Autodesk Fusion 360 part; units mm, degrees
sketch "Skizze2" plane through (0, 0, 0) normal (0, 0, 1) x (1, 0, 0)
  line L0 (15, 50) -> (-15, 50)
  line L1 (-15, 50) -> (-15, -50)
  line L2 (-15, -50) -> (15, -50)
  line L3 (15, -50) -> (15, 50)
  line L4 (15, 50) -> (-15, -50) construction
  line L5 (-15, 50) -> (15, -50) construction
  circle A0 centre (15, 50) radius 2.3
  circle A1 centre (-15, 50) radius 2.3
  circle A2 centre (-15, -50) radius 2.3
  circle A3 centre (15, -50) radius 2.3
  line L6 (40, 86) -> (-40, 86)
  line L7 (-40, 86) -> (-40, -86)
  line L8 (-40, -86) -> (40, -86)
  line L9 (40, -86) -> (40, 86)
  line L10 (40, 86) -> (-40, -86) construction
  line L11 (-40, 86) -> (40, -86) construction
  line L12 (-30, -86) -> (-30, 86)
  line L13 (30, 86) -> (30, -86)
  line L14 (0, 0) -> (0, -50)
  circle A4 centre (-30, -76) radius 2.75
  circle A5 centre (-30, 0) radius 2.75
  circle A6 centre (-30, 76) radius 2.75
  line L15 (-30, 76) -> (30, 76)
  line L16 (-30, 0) -> (30, 0)
  line L17 (-30, -76) -> (30, -76)
  circle A7 centre (30, -76) radius 2.75
  circle A8 centre (30, 0) radius 2.75
  circle A9 centre (30, 76) radius 2.75
  dimension "d1" = 4.6
  dimension "d2" = 30
  dimension "d3" = 100
  dimension "d4" = 36
  dimension "d5" = 80
  dimension "d6" = 60
  dimension "d7" = 10
  dimension "d8" = 10
  dimension "d9" = 5.5
extrude "Extrusion1" add sketch "Skizze2" against normal blind 6 contours L0 L1 L3 A0 A1 L12 L13 A5 A6 L15 L16 A8 A9 | L0 L1 L3 A0 A1 L16 | L1 L2 A2 L14 L16 | L1 L2 L3 A2 A3 L12 L13 A4 A5 L16 L17 A7 A8 | L2 L3 A3 L14 L16 | L6 L7 L8 L12 A4 A5 A6 | L6 L8 L9 L13 A7 A8 A9 | L6 L12 L13 A6 L15 A9 | L8 L12 L13 A4 L17 A7
fillet "Abrundung1" radius 5 4 edges at (40, -86, -3) (-40, -86, -3) (40, 86, -3) (-40, 86, -3)
hole "Bohrung1" at (30, 0, 0) at (30, 76, 0) at (30, -76, 0) at (-30, -76, 0) at (-30, 0, 0) at (-30, 76, 0) direction (0, 0, -1) diameter 5 depth 30 tip angle 118 countersink diameter 10.5 countersink angle 90
equation "d8 = d7"
Could you check a few things on this model? Use its own coordinates, in mm. Coordinates: 2 decimals unless noted, no trailing zeros. Loops run counter-clockwise (first coordinate to the right, second up) from the corner with the lowest first, then second, coordinate; pieces in that order, holes last. Notation, with made-up numbers: M 72.5,50 L 76.5,50 A16 cw 76.5,68 Z; hole C 89.25,88.5 d5. An arc over 180 degrees is marked long. Put each result on its own line as item: value. Start each with the question number.
(1) Suppose I cut it at C-C on x = 15. Please give me the cut outline in (y, z), then the cut area to 3 significant figures.
(2) I need wall thicknesses on line 1 (Y direction, x = 15, z = -1.5); line 2 (Y direction, x = 30, z = -5.2); line 3 (X direction, y = 76, z = -4.55). Which ranges of each line are inside material? Lowest first, please. Write a range as from..to.
(3) Will these pins go through, and if not, where does the flat tip stop? P1, Ø9, axis at x = 30, y = 76, coming from the +Z side; P2, Ø3, axis at x = -15, y = 50, coming from the +Z side; P3, Ø6.5, axis at x = 30, y = 0, coming from the +Z side.
(4) Suppose I cut it at A-A on y = 0. Please give me the cut outline in (x, z), then the cut area to 4 significant figures.
(5) Suppose I cut it at D-D on y = -50. Please give me the cut outline in (x, z).
(6) Suppose I cut it at B-B on z = -1.3. Count the separate pieces of the cut face and the enclosed holes in it, then the cut area to 3 significant figures.
(7) Thinking about a two-plate mould opening in X: for faces 1 (the face through (30.128, -73.096, -2.344)), 2 (the face through (-39, 84, -3)), 3 (the face through (-13.94, -52.04, -2.96)), 4 (the face through (-1, 1, 0)), which applies, pulls with the +X half, pulls with the -X half, needs draft (parallel to the pull), parting line crosses it, or undercut?
Solutions:
1. outline: M -86,-6 L -52.3,-6 L -52.3,0 L -86,0 Z; M -47.7,-6 L 47.7,-6 L 47.7,0 L -47.7,0 Z; M 52.3,-6 L 86,-6 L 86,0 L 52.3,0 Z
1. area: 977 mm2
2. line 1: y = -86..-52.3, -47.7..47.7, 52.3..86
2. line 2: y = -86..-78.75, -73.25..-2.75, 2.75..73.25, 78.75..86
2. line 3: x = -40..-32.75, -27.25..27.25, 32.75..40
3. P1: stops at z = -0.75
3. P2: passes through
3. P3: stops at z = -2
4. outline: M -40,-6 L -32.75,-6 L -32.75,-2.5 L -35.25,0 L -40,0 Z; M -27.25,-6 L 27.25,-6 L 27.25,-2.5 L 24.75,0 L -24.75,0 L -27.25,-2.5 Z; M 32.75,-6 L 40,-6 L 40,0 L 35.25,0 L 32.75,-2.5 Z
4. area: 401.5 mm2
5. outline: M -40,-6 L -17.3,-6 L -17.3,0 L -40,0 Z; M -12.7,-6 L 12.7,-6 L 12.7,0 L -12.7,0 Z; M 17.3,-6 L 40,-6 L 40,0 L 17.3,0 Z
6. separate pieces: 1
6. enclosed holes: 10
6. area: 13,400 mm2
7. face 1: undercut
7. face 2: pulls with the -X half
7. face 3: undercut
7. face 4: needs draft
